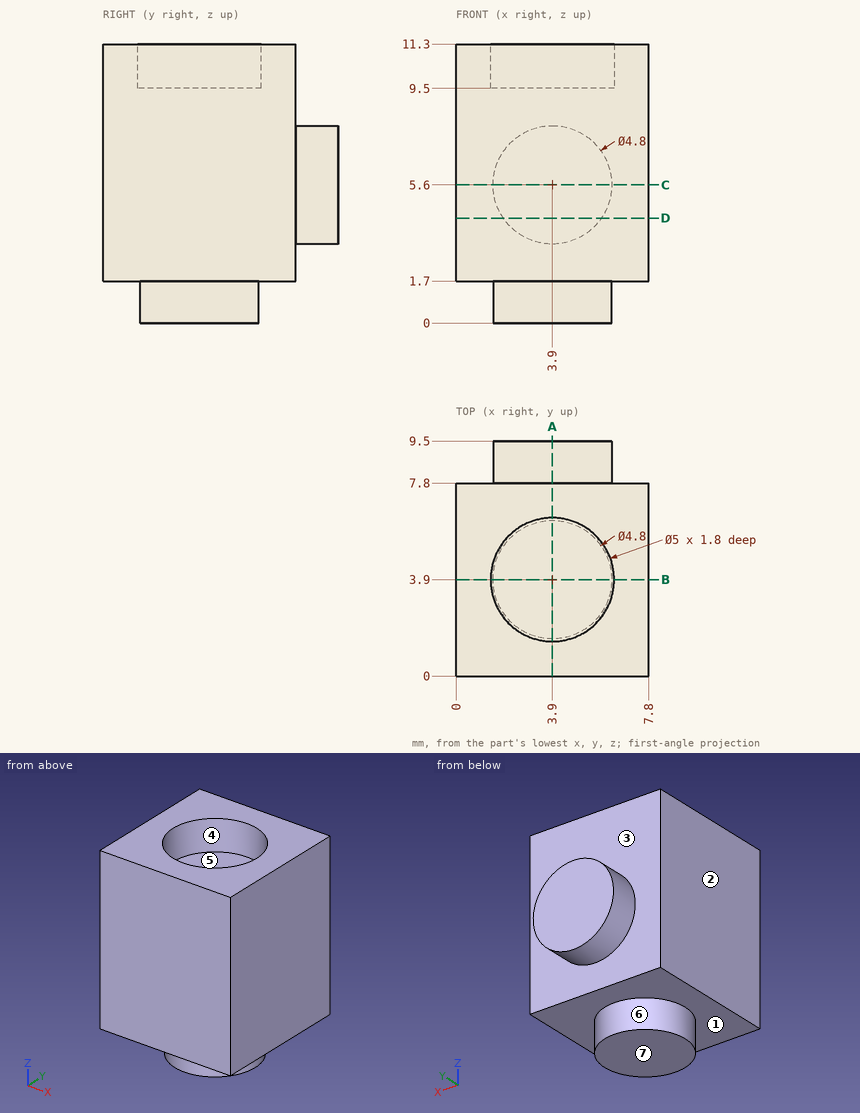
Could you check a few things on this drawing? It's one solid part, dimensions in mm from its lowest x, y, z. A direction names the side the tool comes from. Give positions to 0.01 mm unless a question says otherwise; leave off trailing zeros. Write each loop counter-clockwise with the first axis right and the second up, starting at its lowest first coordinate (ties: lowest second). Pieces come first, ordered by that corner, then holes. Notation, with made-up numbers: (89.25, -3.5) -> (98.25, -3.5) arc R17 cw to (98.25, 20.5) -> close; hole circle Ø1 at (-26, 0.5). An arc over 180 degrees is marked (long way). Answer as a JSON object with one key per item and string values.
Q1. Will these pins go through, and if not, where does the flat tip stop? pin 1 Ø2 at (x, y) = (5, 8.5) entering from -Z; pin 2 Ø2 at (x, z) = (5, 9) entering from +Y.
Taken from the geometry:
{"pin 1": "stops at z = 1.7", "pin 2": "stops at y = 7.8"}
Q2. We'd pull the mould along X, two halves only. Please class the marked faces 4, 5, 6 and 7: released by +X, released by -X, zero draft, split by the parting line, or undercut.
Taken from the geometry:
{"face 4": "undercut", "face 5": "undercut", "face 6": "split by the parting line", "face 7": "zero draft"}
Q3. Please list where these lines run through material, in increasing order: L1, parallel to Y at x = 3.9, z = 10.7; L2, parallel to Z at x = 6.5, y = 3.25; L3, parallel to Z at x = 5.5, y = 4.5.
Taken from the geometry:
{"L1": "y = 0 to 1.4, 6.4 to 7.8", "L2": "z = 1.7 to 11.3", "L3": "z = 0 to 9.5"}
Q4. Which directions (+Z, -Z, +X, -X, +Y, -Y) give clear straight access to the entire face, cutting with the end or side of a thin tool? Please do the marked faces 1, 2 and 3.
Taken from the geometry:
{"face 1": "-Z", "face 2": "+Z, -Z, -X, +Y, -Y", "face 3": "+Y"}
Q5. Suppose I cut it at B-B on y = 3.9. Write out the boundary of the cut face in (x, z), then the cut area to 3 significant figures.
Taken from the geometry:
{"outline": "(0, 1.7) -> (1.5, 1.7) -> (1.5, 0) -> (6.3, 0) -> (6.3, 1.7) -> (7.8, 1.7) -> (7.8, 11.3) -> (6.4, 11.3) -> (6.4, 9.5) -> (1.4, 9.5) -> (1.4, 11.3) -> (0, 11.3) -> close", "area": "74.0 mm²"}
Q6. Suppose I cut it at D-D on z = 4.25. Write out the boundary of the cut face in (x, y), then the cut area to 3 significant figures.
Taken from the geometry:
{"outline": "(0, 0) -> (7.8, 0) -> (7.8, 7.8) -> (5.88, 7.8) -> (5.88, 9.5) -> (1.92, 9.5) -> (1.92, 7.8) -> (0, 7.8) -> close", "area": "67.6 mm²"}
Q7. Suppose I cut it at A-A on x = 3.9. Write out the boundary of the cut face in (y, z).
Taken from the geometry:
{"outline": "(0, 1.7) -> (1.5, 1.7) -> (1.5, 0) -> (6.3, 0) -> (6.3, 1.7) -> (7.8, 1.7) -> (7.8, 3.2) -> (9.5, 3.2) -> (9.5, 8) -> (7.8, 8) -> (7.8, 11.3) -> (6.4, 11.3) -> (6.4, 9.5) -> (1.4, 9.5) -> (1.4, 11.3) -> (0, 11.3) -> close"}
Q8. Suppose I cut it at C-C on z = 5.6. Write out the boundary of the cut face in (x, y).
Taken from the geometry:
{"outline": "(0, 0) -> (7.8, 0) -> (7.8, 7.8) -> (6.3, 7.8) -> (6.3, 9.5) -> (1.5, 9.5) -> (1.5, 7.8) -> (0, 7.8) -> close"}
